CAD build for the part. Positions are in the model's coordinates, mm. A direction names the side the tool comes from. Round coordinates to 2 decimals unless told otherwise and drop trailing zeros. Order: outer loops, then holes, each group sorted by start corner. A loop starts at its lowest first (then second) coordinate and runs counter-clockwise, first axis right, second up. Notation, with made-up numbers: (74.25, -21) -> (85.25, -21) arc R26 cw to (85.25, 2) -> close; hole circle Ø4 at (34, -36.5). An arc over 180 degrees is marked (long way). Return JSON: item names as keys, results as strings. Group by question number.
Q1. Which spindle directions (+Z, -Z, +X, -X, +Y, -Y) get a long thin tool onto all of the face, cutting with end or side? Do faces 4 (the flat face through (83, 25, -9.525)), 5 (the flat face through (82, 25, -6.35)), 6 (the flat face through (-76, 0, -12)). Say none if no direction does.
Q2. Probe line 1 along Z through (x, y) = (0, 39) (3 decimals); line 2 along Z through (x, y) = (-10.5, 3); line 3 along X through (y, z) = (9, 51). List the from-to ranges inside material, lowest first.
Q3. Cut at A-A (x = 0). Write the cut outline in (y, z) (3 decimals), then the cut area to 3 significant figures.
Q4. Cut at B-B (y = 35.5). Write the cut outline in (x, z) (3 decimals), then the cut area to 3 significant figures.
Q5. Flat gauge pins, fed straight in: pin 1 (3 mm diameter, centred on y = 29.5, z = -42, fed in from +X); pin 2 (2 mm diameter, centred on x = 68, y = 43.5, fed in from -Z); pin 3 (12 mm diameter, centred on x = 57.5, z = 52.5, fed in from -Y); pin 4 (4 mm diameter, centred on x = 50.5, y = 27.5, fed in from +Z). Where does each tip first touch, or does it go through?
Q6. Mould opens along Z. For faces 1 (the flat face through (83, 25, 9.525)), 2 (the cylindrical face through (-76.13, 25.04, -3.26)), 3 (the flat face through (-76, 50.8, -12)) say: +Z half, -Z half, draft (parallel to the pull), parting line (faces both ways), or undercut.
Q7. Cut at C-C (z = -48). Write the cut outline in (x, y).
Q8. Cut at D-D (z = 0). Write the cut outline in (x, y) (3 decimals), then the cut area to 3 significant figures.
from build123d import *

# Parameters (mm, degrees)
BOSS_EXTRUDE1_DEPTH = 50.8


with BuildPart() as part:
    # Sketch2 → Boss-Extrude1 (new body)
    with BuildSketch(Plane(origin=(0, 0, 0), x_dir=(1, 0, 0), z_dir=(0, 1, 0))):
        with BuildLine():
            Line((78.800950314, -6.35), (87.690950314, -6.35))
            Line((87.690950314, -6.35), (87.690950314, -9.525))
            Line((87.690950314, -9.525), (78.801427652, -9.525))
            ThreePointArc((78.801427652, -9.525), (-79.375, 0), (78.801427652, 9.525))
            Line((78.801427652, 9.525), (87.690950314, 9.525))
            Line((87.690950314, 9.525), (87.690950314, 6.35))
            Line((87.690950314, 6.35), (78.800950314, 6.35))
            Line((78.800950314, 6.35), (75.934955719, 6.35))
            ThreePointArc((75.934955719, 6.35), (-76.2, 0), (75.934955719, -6.35))
            Line((75.934955719, -6.35), (78.800950314, -6.35))
        make_face()
    extrude(amount=BOSS_EXTRUDE1_DEPTH)


solid = part.part
Solution:
{
 "1": {"face 4": "-Z, +X, +Y, -Y", "face 5": "+X, +Y, -Y", "face 6": "+Z, -Z, +X, -X, -Y"},
 "2": {"line 1": "z = -79.375 to -76.2, 76.2 to 79.375", "line 2": "z = -78.68 to -75.47, 75.47 to 78.68", "line 3": "x = -60.82 to -56.62, 56.62 to 60.82"},
 "3": {"outline": "(0, -79.375) -> (50.8, -79.375) -> (50.8, -76.2) -> (0, -76.2) -> close; (0, 76.2) -> (50.8, 76.2) -> (50.8, 79.375) -> (0, 79.375) -> close", "area": "323 mm²"},
 "4": {"outline": "(75.935, -6.35) arc R76.2 cw (long way) to (75.935, 6.35) -> (87.691, 6.35) -> (87.691, 9.525) -> (78.801, 9.525) arc R79.375 ccw (long way) to (78.801, -9.525) -> (87.691, -9.525) -> (87.691, -6.35) -> close", "area": "1,570 mm²"},
 "5": {"pin 1": "stops at x = 68.27", "pin 2": "stops at z = -42.56", "pin 3": "stops at y = 0", "pin 4": "stops at z = 62.83"},
 "6": {"face 1": "+Z half", "face 2": "undercut", "face 3": "draft"},
 "7": {"outline": "(-63.22, 0) -> (-59.18, 0) -> (-59.18, 50.8) -> (-63.22, 50.8) -> close; (59.18, 0) -> (63.22, 0) -> (63.22, 50.8) -> (59.18, 50.8) -> close"},
 "8": {"outline": "(-79.375, 0) -> (-76.2, 0) -> (-76.2, 50.8) -> (-79.375, 50.8) -> close", "area": "161 mm²"}
}
